The listing builds one solid part. Answer for the finished solid, in the listing's coordinates (mm). Face numbers are marked on the shaded views. A direction names the side the tool comes from. Give positions to 0.01 mm unless a question says otherwise; leave off trailing zeros. Write each loop counter-clockwise with the first axis right and the second up, starting at its lowest first coordinate (ties: lowest second). Pieces come first, ordered by that corner, then holes. Notation, with made-up numbers: (-1.5, 73.5) - (19.5, 73.5) arc R26 ccw to (19.5, 92.5) - close; hole circle Ø8 at (64.25, -21.75). An arc over 180 degrees is marked (long way). One line per item, written item: value. Start each with the question number.
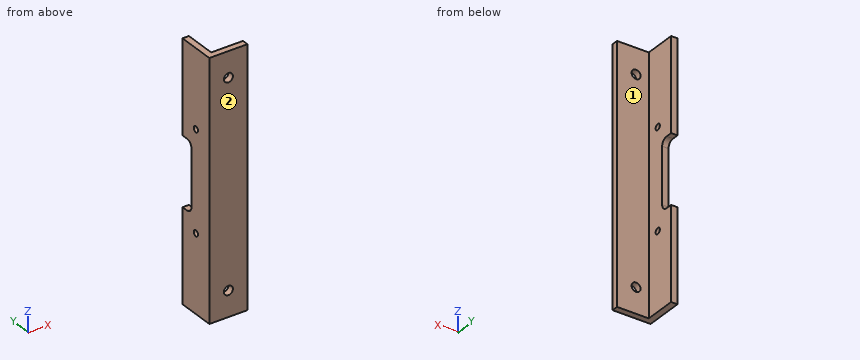
from build123d import *

# Parameters (mm, degrees)
F1_DEPTH  = 254
F3_D      = 9
F4_D      = 9
F9_D      = 6
F11_DEPTH = 6.35


with BuildPart() as f1:
    # F0 (on Top) → F1 (new body)
    with BuildSketch(Plane.XY):
        Polygon((0, 38.1), (0, 0), (38.1, 0), (38.1, 6.35), (6.35, 6.35), (6.35, 38.1), align=None)
    extrude(amount=F1_DEPTH)

    # F3 (through all)
    with Locations(Plane.XZ):
        with Locations((19.05, 228.6)):
            Hole(F3_D / 2)

    # F4 (through all)
    with Locations(Plane.XZ):
        with Locations((19.05, 25.4)):
            Hole(F4_D / 2)

    # F9 (through all)
    with Locations(Plane(origin=(0, 0, 0), x_dir=(0, -1, 0), z_dir=(-1, 0, 0))):
        with Locations((-19.05, 77.216), (-19.05, 176.53)):
            Hole(F9_D / 2)

    # F10 (on face) → F11 (cut, through all)
    with BuildSketch(Plane.YZ.offset(6.35)):
        with BuildLine():
            ThreePointArc((31.75, 161.29), (27.259872, 159.430128), (25.4, 154.94))
            Line((25.4, 154.94), (25.4, 99.06))
            ThreePointArc((25.4, 99.06), (27.259872, 94.569872), (31.75, 92.71))
            Line((31.75, 92.71), (38.1, 92.71))
            Line((38.1, 92.71), (38.1, 161.29))
            Line((38.1, 161.29), (31.75, 161.29))
        make_face()
    extrude(amount=-F11_DEPTH, mode=Mode.SUBTRACT)


solid = f1.part
Item 1: Find section D-D on x = 4. Determine the outline of the cut face in (y, z).
Item 2: Find section B-B on y = 19.05. Determine the outline of the cut face in (x, z), plus the area to 3 significant figures.
Item 3: Each of these flat-tipped pins is pushed along its axis until it touches: pin 1 Ø7 at (x, z) = (2.5, 116) entering from +Y; pin 2 Ø9.5 at (y, z) = (14.5, 148.5) entering from +X; pin 3 Ø3.5 at (y, z) = (19.05, 176.53) entering from -X; pin 4 Ø9.5 at (x, z) = (26.5, 156) entering from +Y. Where does it stop, or does it pass through?
Item 4: Find section C-C on x = 19.05. Determine the outline of the cut face in (y, z), plus the area to 3 significant figures.
Item 5: Straight lines are drawn through the part: line 1 along Z through (x, y) = (4, 19); line 2 along Z through (x, y) = (19.05, 2.25); line 3 along Z through (x, y) = (6, 34). For each, find the intervals that lie inside material, in ascending order.
Item 6: Find section A-A on z = 176.53. Determine the outline of the cut face in (x, y), plus the area to 3 significant figures.
Item 7: For the marked faces 1 and 2, determine the directions among +Z, -Z, +X, -X, +Y, -Y from which every point of the face is accessible in a straight line to the end or side of a thin tool.
Values:
1. outline: (0, 0) - (38.1, 0) - (38.1, 92.71) - (31.75, 92.71) arc R6.35 cw to (25.4, 99.06) - (25.4, 154.94) arc R6.35 cw to (31.75, 161.29) - (38.1, 161.29) - (38.1, 254) - (0, 254) - close; hole circle Ø6 at (19.05, 77.22); hole circle Ø6 at (19.05, 176.53)
2. outline: (0, 0) - (6.35, 0) - (6.35, 74.22) - (0, 74.22) - close; (0, 80.22) - (6.35, 80.22) - (6.35, 173.53) - (0, 173.53) - close; (0, 179.53) - (6.35, 179.53) - (6.35, 254) - (0, 254) - close
2. area: 1,540 mm^2
3. pin 1: y = 25.4
3. pin 2: x = 6.35
3. pin 3: through
3. pin 4: y = 6.35
4. outline: (0, 0) - (6.35, 0) - (6.35, 20.9) - (0, 20.9) - close; (0, 29.9) - (6.35, 29.9) - (6.35, 224.1) - (0, 224.1) - close; (0, 233.1) - (6.35, 233.1) - (6.35, 254) - (0, 254) - close
4. area: 1,500 mm^2
5. line 1: 0 to 74.22, 80.22 to 173.53, 179.53 to 254
5. line 2: 0 to 20.9, 29.9 to 224.1, 233.1 to 254
5. line 3: 0 to 92.71, 161.29 to 254
6. outline: (0, 0) - (38.1, 0) - (38.1, 6.35) - (6.35, 6.35) - (6.35, 16.05) - (0, 16.05) - close; (0, 22.05) - (6.35, 22.05) - (6.35, 38.1) - (0, 38.1) - close
6. area: 405 mm^2
7. face 1: +Z, -Z, +X, +Y
7. face 2: +Z, -Z, +X, -X, -Y
